```python
from build123d import *

# Parameters (mm, degrees)
BOSS_EXTRUDE1_DEPTH = 14.8
BOSS_EXTRUDE2_DEPTH = 2
FILLET1_R           = 4


with BuildPart() as part:
    # Sketch1 → Boss-Extrude1 (new body)
    with BuildSketch(Plane.XY):
        with BuildLine():
            ThreePointArc((-29.158352439, 21.804727646), (-31.501498189, 16.147873397), (-37.158352439, 13.804727646))
            Line((-37.158352439, 13.804727646), (-37.158352439, -10.195272354))
            ThreePointArc((-37.158352439, -10.195272354), (-31.501498189, -12.538418104), (-29.158352439, -18.195272354))
            Line((-29.158352439, -18.195272354), (19.841647561, -18.195272354))
            ThreePointArc((19.841647561, -18.195272354), (22.184793312, -12.538418104), (27.841647561, -10.195272354))
            Line((27.841647561, -10.195272354), (27.841647561, 13.804727646))
            ThreePointArc((27.841647561, 13.804727646), (22.184793312, 16.147873397), (19.841647561, 21.804727646))
            Line((19.841647561, 21.804727646), (-29.158352439, 21.804727646))
        make_face()
    extrude(amount=BOSS_EXTRUDE1_DEPTH)

    # Sketch1_3 → Boss-Extrude2 (add)
    with BuildSketch(Plane.XY):
        with BuildLine():
            Line((27.841647561, 21.804727646), (19.841647561, 21.804727646))
            ThreePointArc((19.841647561, 21.804727646), (22.184793312, 16.147873397), (27.841647561, 13.804727646))
            Line((27.841647561, 13.804727646), (27.841647561, 21.804727646))
        make_face()
        with BuildLine():
            Line((-29.158352439, 21.804727646), (-37.158352439, 21.804727646))
            Line((-37.158352439, 21.804727646), (-37.158352439, 13.804727646))
            ThreePointArc((-37.158352439, 13.804727646), (-31.501498189, 16.147873397), (-29.158352439, 21.804727646))
        make_face()
        with BuildLine():
            ThreePointArc((27.841647561, -10.195272354), (22.184793312, -12.538418104), (19.841647561, -18.195272354))
            Line((19.841647561, -18.195272354), (27.841647561, -18.195272354))
            Line((27.841647561, -18.195272354), (27.841647561, -10.195272354))
        make_face()
        with BuildLine():
            ThreePointArc((-29.158352439, -18.195272354), (-31.501498189, -12.538418104), (-37.158352439, -10.195272354))
            Line((-37.158352439, -10.195272354), (-37.158352439, -18.195272354))
            Line((-37.158352439, -18.195272354), (-29.158352439, -18.195272354))
        make_face()
        with BuildLine():
            ThreePointArc((-29.158352439, 21.804727646), (-31.501498189, 16.147873397), (-37.158352439, 13.804727646))
            Line((-37.158352439, 13.804727646), (-37.158352439, -10.195272354))
            ThreePointArc((-37.158352439, -10.195272354), (-31.501498189, -12.538418104), (-29.158352439, -18.195272354))
            Line((-29.158352439, -18.195272354), (19.841647561, -18.195272354))
            ThreePointArc((19.841647561, -18.195272354), (22.184793312, -12.538418104), (27.841647561, -10.195272354))
            Line((27.841647561, -10.195272354), (27.841647561, 13.804727646))
            ThreePointArc((27.841647561, 13.804727646), (22.184793312, 16.147873397), (19.841647561, 21.804727646))
            Line((19.841647561, 21.804727646), (-29.158352439, 21.804727646))
        make_face()
    extrude(amount=-BOSS_EXTRUDE2_DEPTH)

    # Fillet1
    fillet1_edges = [part.edges().sort_by_distance(p)[0] for p in [
        (22.184793312, 16.147873397, 14.8),
        (-4.658352439, 21.804727646, 14.8),
        (-31.501498189, 16.147873397, 14.8),
        (-37.158352439, 1.804727646, 14.8),
        (-31.501498189, -12.538418104, 14.8),
        (-4.658352439, -18.195272354, 14.8),
        (22.184793312, -12.538418104, 14.8),
        (27.841647561, 1.804727646, 14.8),
    ]]
    fillet(fillet1_edges, radius=FILLET1_R)


solid = part.part
```
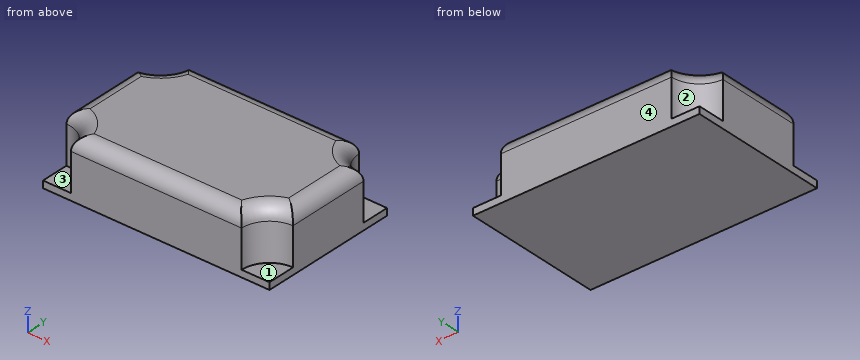
Input: part model. Units: mm. Frame: model coordinates. Face numbers are marked on the shaded views. A direction names the side the tool comes from. Give positions to 0.01 mm unless a question says otherwise; leave off trailing zeros. Order: outer loops, then holes, each group sorted by start corner. A loop starts at its lowest first (then second) coordinate and runs counter-clockwise, first axis right, second up. Notation, with made-up numbers: (-28, 69.5) -> (16, 69.5) arc R28 cw to (16, 99.5) -> close; hole circle Ø6 at (-23.5, 71). An arc over 180 degrees is marked (long way). Write each question's results on one line, items separated by ' | '. Start each with the question number.
Item 1: Cut plane A-A on z = 6. Return the cut outline in (x, y).
Item 2: Contact query for flat-ended pins moving along their axis: P1, Ø6.5, axis at x = -31.5, y = 18.5, coming from the +Z side; P2, Ø6.5, axis at x = -33, y = -13.5, coming from the +Z side; P3, Ø6.5, axis at x = 23, y = 17, coming from the +Z side. Output: stop coordinate, or through.
Item 3: Line query: line 1 (Y direction, x = -33, z = 10.25); line 2 (Y direction, x = 9, z = 13.75); line 3 (X direction, y = 16, z = 12.75). Output: solid intervals per line, ascending.
Item 4: Set-up query: the marked faces 1, 2, 3 and 4. Return all of +Z, -Z, +X, -X, +Y, -Y with unobstructed straight access to the full face (end or side cutting, diameter ignored); none if empty.
Established:
1) outline: (-37.16, -10.2) arc R8 cw to (-29.16, -18.2) -> (19.84, -18.2) arc R8 cw to (27.84, -10.2) -> (27.84, 13.8) arc R8 cw to (19.84, 21.8) -> (-29.16, 21.8) arc R8 cw to (-37.16, 13.8) -> close
2) P1: z = 14.14 | P2: z = 13.94 | P3: z = 14.3
3) line 1: -11.36 to 14.97 | line 2: -16.9 to 20.51 | line 3: -30.94 to 21.62
4) face 1: +Z, +X, -Y | face 2: +Z, -X, +Y | face 3: +Z, -X, -Y | face 4: +Z, -Z, +X, -X, +Y
